Build history of the part. All positions in model axes, mm. A direction names the side the tool comes from. Give positions to 0.01 mm unless a question says otherwise; leave off trailing zeros. Write each loop counter-clockwise with the first axis right and the second up, starting at its lowest first coordinate (ties: lowest second). Pieces come first, ordered by that corner, then holes. Notation, with made-up numbers: (-35, 43) - (-10, 43) arc R14 ccw to (-10, 60) - close; hole circle Ø3 at (-18.5, 16). An arc over 180 degrees is marked (long way). Use one line per item in the form item = value. Start each with the question number.
from build123d import *

# Parameters (mm, degrees)
BOSS_EXTRUDE1_DEPTH = 1219.2
SKETCH3_R           = 4.7625
CUT_EXTRUDE1_DEPTH  = 1.27
SKETCH4_R           = 4.7625
CUT_EXTRUDE2_DEPTH  = 1.27
FILLET1_R           = 3.175
FILLET2_R           = 1.5875


with BuildPart() as part:
    # Sketch1 → Boss-Extrude1 (new body)
    with BuildSketch(Plane(origin=(0, 0, 0), x_dir=(1, 0, 0), z_dir=(0, 1, 0))):
        Polygon((1.27, 1.27), (1.27, 30.48), (1.27, 31.75), (0, 31.75), (0, 0), (31.75, 0), (31.75, 1.27), (30.48, 1.27), align=None)
    extrude(amount=BOSS_EXTRUDE1_DEPTH)

    # Sketch3 → Cut-Extrude1 (cut)
    with BuildSketch(Plane.ZY):
        with Locations((-15.875, 12.7)):
            Circle(SKETCH3_R)
        with Locations((-15.875, 38.1)):
            Circle(SKETCH3_R)
        with Locations((-15.875, 63.5)):
            Circle(SKETCH3_R)
        with Locations((-15.875, 88.9)):
            Circle(SKETCH3_R)
        with Locations((-15.875, 114.3)):
            Circle(SKETCH3_R)
        with Locations((-15.875, 139.7)):
            Circle(SKETCH3_R)
        with Locations((-15.875, 165.1)):
            Circle(SKETCH3_R)
        with Locations((-15.875, 190.5)):
            Circle(SKETCH3_R)
        with Locations((-15.875, 215.9)):
            Circle(SKETCH3_R)
        with Locations((-15.875, 241.3)):
            Circle(SKETCH3_R)
        with Locations((-15.875, 266.7)):
            Circle(SKETCH3_R)
        with Locations((-15.875, 292.1)):
            Circle(SKETCH3_R)
        with Locations((-15.875, 317.5)):
            Circle(SKETCH3_R)
        with Locations((-15.875, 342.9)):
            Circle(SKETCH3_R)
        with Locations((-15.875, 368.3)):
            Circle(SKETCH3_R)
        with Locations((-15.875, 393.7)):
            Circle(SKETCH3_R)
        with Locations((-15.875, 419.1)):
            Circle(SKETCH3_R)
        with Locations((-15.875, 444.5)):
            Circle(SKETCH3_R)
        with Locations((-15.875, 469.9)):
            Circle(SKETCH3_R)
        with Locations((-15.875, 495.3)):
            Circle(SKETCH3_R)
        with Locations((-15.875, 520.7)):
            Circle(SKETCH3_R)
        with Locations((-15.875, 546.1)):
            Circle(SKETCH3_R)
        with Locations((-15.875, 571.5)):
            Circle(SKETCH3_R)
        with Locations((-15.875, 596.9)):
            Circle(SKETCH3_R)
        with Locations((-15.875, 622.3)):
            Circle(SKETCH3_R)
        with Locations((-15.875, 647.7)):
            Circle(SKETCH3_R)
        with Locations((-15.875, 673.1)):
            Circle(SKETCH3_R)
        with Locations((-15.875, 698.5)):
            Circle(SKETCH3_R)
        with Locations((-15.875, 723.9)):
            Circle(SKETCH3_R)
        with Locations((-15.875, 749.3)):
            Circle(SKETCH3_R)
        with Locations((-15.875, 774.7)):
            Circle(SKETCH3_R)
        with Locations((-15.875, 800.1)):
            Circle(SKETCH3_R)
        with Locations((-15.875, 825.5)):
            Circle(SKETCH3_R)
        with Locations((-15.875, 850.9)):
            Circle(SKETCH3_R)
        with Locations((-15.875, 876.3)):
            Circle(SKETCH3_R)
        with Locations((-15.875, 901.7)):
            Circle(SKETCH3_R)
        with Locations((-15.875, 927.1)):
            Circle(SKETCH3_R)
        with Locations((-15.875, 952.5)):
            Circle(SKETCH3_R)
        with Locations((-15.875, 977.9)):
            Circle(SKETCH3_R)
        with Locations((-15.875, 1003.3)):
            Circle(SKETCH3_R)
        with Locations((-15.875, 1028.7)):
            Circle(SKETCH3_R)
        with Locations((-15.875, 1054.1)):
            Circle(SKETCH3_R)
        with Locations((-15.875, 1079.5)):
            Circle(SKETCH3_R)
        with Locations((-15.875, 1104.9)):
            Circle(SKETCH3_R)
        with Locations((-15.875, 1130.3)):
            Circle(SKETCH3_R)
        with Locations((-15.875, 1155.7)):
            Circle(SKETCH3_R)
        with Locations((-15.875, 1181.1)):
            Circle(SKETCH3_R)
        with Locations((-15.875, 1206.5)):
            Circle(SKETCH3_R)
    extrude(amount=-CUT_EXTRUDE1_DEPTH, mode=Mode.SUBTRACT)

    # Sketch4 → Cut-Extrude2 (cut)
    with BuildSketch(Plane.XY):
        with Locations((15.875, 1206.5)):
            Circle(SKETCH4_R)
        with Locations((15.875, 1181.1)):
            Circle(SKETCH4_R)
        with Locations((15.875, 1155.7)):
            Circle(SKETCH4_R)
        with Locations((15.875, 1130.3)):
            Circle(SKETCH4_R)
        with Locations((15.875, 1104.9)):
            Circle(SKETCH4_R)
        with Locations((15.875, 1079.5)):
            Circle(SKETCH4_R)
        with Locations((15.875, 1054.1)):
            Circle(SKETCH4_R)
        with Locations((15.875, 1028.7)):
            Circle(SKETCH4_R)
        with Locations((15.875, 1003.3)):
            Circle(SKETCH4_R)
        with Locations((15.875, 977.9)):
            Circle(SKETCH4_R)
        with Locations((15.875, 952.5)):
            Circle(SKETCH4_R)
        with Locations((15.875, 927.1)):
            Circle(SKETCH4_R)
        with Locations((15.875, 901.7)):
            Circle(SKETCH4_R)
        with Locations((15.875, 876.3)):
            Circle(SKETCH4_R)
        with Locations((15.875, 850.9)):
            Circle(SKETCH4_R)
        with Locations((15.875, 825.5)):
            Circle(SKETCH4_R)
        with Locations((15.875, 800.1)):
            Circle(SKETCH4_R)
        with Locations((15.875, 774.7)):
            Circle(SKETCH4_R)
        with Locations((15.875, 749.3)):
            Circle(SKETCH4_R)
        with Locations((15.875, 723.9)):
            Circle(SKETCH4_R)
        with Locations((15.875, 698.5)):
            Circle(SKETCH4_R)
        with Locations((15.875, 673.1)):
            Circle(SKETCH4_R)
        with Locations((15.875, 647.7)):
            Circle(SKETCH4_R)
        with Locations((15.875, 622.3)):
            Circle(SKETCH4_R)
        with Locations((15.875, 596.9)):
            Circle(SKETCH4_R)
        with Locations((15.875, 571.5)):
            Circle(SKETCH4_R)
        with Locations((15.875, 546.1)):
            Circle(SKETCH4_R)
        with Locations((15.875, 520.7)):
            Circle(SKETCH4_R)
        with Locations((15.875, 495.3)):
            Circle(SKETCH4_R)
        with Locations((15.875, 469.9)):
            Circle(SKETCH4_R)
        with Locations((15.875, 444.5)):
            Circle(SKETCH4_R)
        with Locations((15.875, 419.1)):
            Circle(SKETCH4_R)
        with Locations((15.875, 393.7)):
            Circle(SKETCH4_R)
        with Locations((15.875, 368.3)):
            Circle(SKETCH4_R)
        with Locations((15.875, 342.9)):
            Circle(SKETCH4_R)
        with Locations((15.875, 317.5)):
            Circle(SKETCH4_R)
        with Locations((15.875, 292.1)):
            Circle(SKETCH4_R)
        with Locations((15.875, 266.7)):
            Circle(SKETCH4_R)
        with Locations((15.875, 241.3)):
            Circle(SKETCH4_R)
        with Locations((15.875, 215.9)):
            Circle(SKETCH4_R)
        with Locations((15.875, 190.5)):
            Circle(SKETCH4_R)
        with Locations((15.875, 165.1)):
            Circle(SKETCH4_R)
        with Locations((15.875, 139.7)):
            Circle(SKETCH4_R)
        with Locations((15.875, 114.3)):
            Circle(SKETCH4_R)
        with Locations((15.875, 88.9)):
            Circle(SKETCH4_R)
        with Locations((15.875, 63.5)):
            Circle(SKETCH4_R)
        with Locations((15.875, 38.1)):
            Circle(SKETCH4_R)
        with Locations((15.875, 12.7)):
            Circle(SKETCH4_R)
    extrude(amount=-CUT_EXTRUDE2_DEPTH, mode=Mode.SUBTRACT)

    # Fillet1
    fillet1_edges = [part.edges().sort_by_distance(p)[0] for p in [
        (0, 609.6, 0),
    ]]
    fillet(fillet1_edges, radius=FILLET1_R)

    # Fillet2
    fillet2_edges = [part.edges().sort_by_distance(p)[0] for p in [
        (1.27, 609.6, -1.27),
    ]]
    fillet(fillet2_edges, radius=FILLET2_R)


solid = part.part
(1) Wall check: line 1 (X direction, y = 749.3, z = -0.65); line 2 (X direction, y = 250, z = -5.5); line 3 (Z direction, x = 18.5, y = 667.5). Give the ranges that are in metal, low to high. Write a range as from..to.
(2) Cut at A-A, the plane x = 26. Give the cut face in (y, z).
(3) Pin check, flat tips, straight feed: pin 1 Ø5.5 at (y, z) = (1206.5, -15.875) entering from -X; pin 2 Ø11 at (x, y) = (15.875, 368.3) entering from -Z; pin 3 Ø1.5 at (y, z) = (1076.5, -21) entering from +X. Stop position of each tip, or through.
(4) Which spindle directions (+Z, -Z, +X, -X, +Y, -Y) get a long thin tool onto all of the face, cutting with end or side? Do faces 1 (the flat face through (1.27, 601, -20)), 2 (the flat face through (1, 1219.2, -9)). Say none if no direction does.
Solution:
q1.line_1 = 1.25..11.11, 20.64..31.75
q1.line_2 = 0..1.27
q1.line_3 = -1.27..0
q2.outline = (0, -1.27) - (1219.2, -1.27) - (1219.2, 0) - (0, 0) - close
q3.pin_1 = through
q3.pin_2 = -1.27
q3.pin_3 = 1.27
q4.face_1 = -Z, +X, +Y, -Y
q4.face_2 = +Z, -Z, +X, -X, +Y
